```python
from build123d import *

# Parameters (mm, degrees)
PAD_DEPTH       = 4
SKETCH001_R     = 115
POCKET_DEPTH    = 10
PAD001_DEPTH    = 2
SKETCH003_R     = 113
POCKET001_DEPTH = 5


with BuildPart() as part:
    # Sketch → Pad (new body)
    with BuildSketch(Plane.XY):
        with BuildLine():
            ThreePointArc((60, -126.491106), (0, 140), (-60, -126.491106))
            ThreePointArc((-40, -150), (-47.476432, -136.098648), (-60, -126.491106))
            ThreePointArc((-40, -150), (0, -180.057233), (40, -150))
            ThreePointArc((60, -126.491106), (47.476432, -136.098648), (40, -150))
        make_face()
    extrude(amount=PAD_DEPTH)

    # Sketch001 → Pocket (cut)
    with BuildSketch(Plane.XY):
        Circle(SKETCH001_R)
    extrude(amount=POCKET_DEPTH, mode=Mode.SUBTRACT)

    # Sketch002 → Pad001 (join)
    with BuildSketch(Plane.XY):
        with BuildLine():
            ThreePointArc((62, -127.749755), (0, 142), (-62, -127.749755))
            ThreePointArc((-42, -152), (-49.356513, -137.694705), (-62, -127.749755))
            ThreePointArc((-42, -152), (0, -184.276954), (42, -152))
            ThreePointArc((62, -127.749755), (49.356513, -137.694705), (42, -152))
        make_face()
    extrude(amount=PAD001_DEPTH)

    # Sketch003 → Pocket001 (cut)
    with BuildSketch(Plane.XY):
        Circle(SKETCH003_R)
    extrude(amount=POCKET001_DEPTH, mode=Mode.SUBTRACT)


solid = part.part
```
Work out the finished part from the listing and answer in its coordinate system (mm). A direction names the side the tool comes from. Round coordinates to 2 decimals unless told otherwise and drop trailing zeros. Loops run counter-clockwise (first coordinate to the right, second up) from the corner with the lowest first, then second, coordinate; pieces in that order, holes last. Notation, with made-up numbers: (-36, 51) -> (11, 51) arc R12 ccw to (11, 59) -> close; hole circle Ø7 at (3, 80.5). An arc over 180 degrees is marked (long way). Write each question's results on one line, items separated by ' | '. Start each with the question number.
1. Given pin 1 Ø1.5 at (y, z) = (-53, 3.5) entering from +X, flat-ended and moving along its own axis, determine where the tip first touches the part or whether it passes through.
2. Section A-A (x = 0) is taken. Determine the outline of the cut face in (y, z).
3. A tool of negligible diameter and unlimited length cuts with its end or side. For faces 1 (the face through (-49.213, -137.87, 0.986)), 2 (the face through (85, -76, 2)), from which of +Z, -Z, +X, -X, +Y, -Y can it reach the whole face along a straight path? Write none if from no direction.
4. Find the intervals of material crossed by probe 1 along X at (y, z) = (0, 3.5); probe 2 along X at (y, z) = (0, 0.8); probe 3 along Y at (x, z) = (0, 2.5), in increasing order. Write a range as from..to.
5. Section C-C (z = 1.3) is taken. Determine the outline of the cut face in (x, y).
6. For a pull along X with two mould halves and no side action, classify faces 3 (the face through (-47.33, -136.27, 2.99)), 4 (the face through (-24.93, -112.265, 2.986)), 5 (the face through (47.62, -135.93, 2.99)), 6 (the face through (-0.75, -180.05, 2.99)) as +X half, -X half, draft (parallel to the pull), parting line (faces both ways), or undercut.
7. Section B-B (y = 0) is taken. Determine the outline of the cut face in (x, z), plus the area to 3 significant figures.
Evaluation:
1) pin 1: stops at x = 129.88
2) outline: (-184.28, 0) -> (-113, 0) -> (-113, 2) -> (-115, 2) -> (-115, 4) -> (-180.06, 4) -> (-180.06, 2) -> (-184.28, 2) -> close; (113, 0) -> (142, 0) -> (142, 2) -> (140, 2) -> (140, 4) -> (115, 4) -> (115, 2) -> (113, 2) -> close
3) face 1: +Z, -Z, -X, -Y | face 2: +Z
4) probe 1: x = -140..-115, 115..140 | probe 2: x = -142..-113, 113..142 | probe 3: y = -180.06..-115, 115..140
5) outline: (-62, -127.75) arc R37.76 cw to (-42, -152) arc R43.46 ccw to (42, -152) arc R37.76 cw to (62, -127.75) arc R142 ccw (long way) to start; hole circle Ø226 at (0, 0)
6) face 3: -X half | face 4: undercut | face 5: +X half | face 6: parting line
7) outline: (-142, 0) -> (-113, 0) -> (-113, 2) -> (-115, 2) -> (-115, 4) -> (-140, 4) -> (-140, 2) -> (-142, 2) -> close; (113, 0) -> (142, 0) -> (142, 2) -> (140, 2) -> (140, 4) -> (115, 4) -> (115, 2) -> (113, 2) -> close | area: 216 mm2
